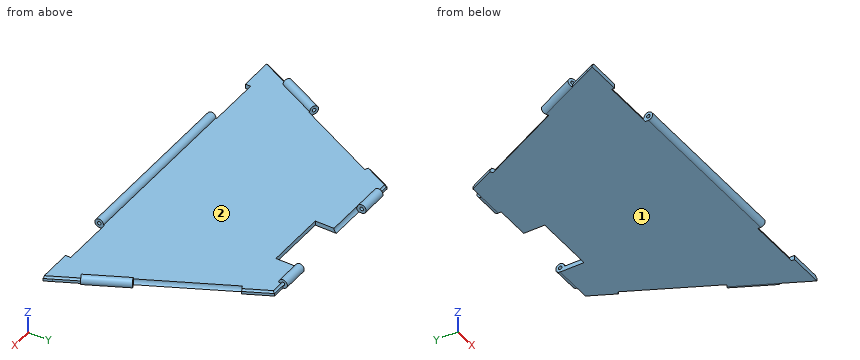
from build123d import *

# Parameters (mm, degrees)
EXTRUDE_1_DEPTH      = 5
SKETCH_9_W           = 30
SKETCH_9_H           = 5
SKETCH_10_R          = 2
CUT_EXTRUDE_3_DEPTH  = 352.212186577
SKETCH_4_W           = 5
SKETCH_4_H           = 50
SKETCH_11_R          = 2
CUT_EXTRUDE_4_DEPTH  = 338.069639722
SKETCH_12_R          = 6
CUT_EXTRUDE_5_DEPTH  = 105
SKETCH_14_R          = 6
CUT_EXTRUDE_6_DEPTH  = 110
SKETCH_3_W           = 200
SKETCH_3_H           = 5
SKETCH_15_R          = 2
CUT_EXTRUDE_7_DEPTH  = 200
SKETCH_16_R          = 6
CUT_EXTRUDE_8_DEPTH  = 60
CUT_EXTRUDE_START    = 60
SKETCH_17_R          = 6
CUT_EXTRUDE_9_DEPTH  = 60
SCALE_1_SCALE        = 0.5
SKETCH_19_W          = 35
SKETCH_19_H          = 12
CUT_EXTRUDE_11_DEPTH = 10


with BuildPart() as part:
    # 草图2 → 凸台-拉伸1 (new body)
    with BuildSketch(Plane(origin=(0, 65.305030884, 0), x_dir=(1, 0, 0), z_dir=(0, 0, 1))):
        Polygon((-200, 0), (-155, 0), (-105, 0), (105, 0), (155, 0), (200, 0), (195.839393539, 8.321212923), (151.118033989, 97.763932023), (100, 200), (50, 200), (-50, 200), (-100, 200), (-151.118033989, 97.763932023), (-195.839393539, 8.321212923), align=None)
    extrude(amount=EXTRUDE_1_DEPTH)

    # 草图9 → 旋转1 (revolve)
    with BuildSketch(Plane(origin=(0, 65.305030884, 5), x_dir=(1, 0, 0), z_dir=(0, 0, 1))):
        with Locations((-70, 197.5)):
            Rectangle(SKETCH_9_W, SKETCH_9_H)
    revolve_1 = revolve(axis=Axis((-85, 265.305030884, 5), (1, 0, 0)))

    # 草图10 → 切除-拉伸3 (cut, symmetric)
    with BuildSketch(Plane(origin=(-85, 65.305030884, 0), x_dir=(0, 0, 1), z_dir=(-1, 0, 0))):
        with Locations(Location((5, 200, 0), (0, 0, 270))):
            Circle(SKETCH_10_R)
    cut_extrude_3 = extrude(amount=CUT_EXTRUDE_3_DEPTH, both=True, mode=Mode.SUBTRACT)

    # 镜向2: 旋转1, 切除-拉伸3 across plane
    add(revolve_1.mirror(Plane(origin=(0, 0, 0), x_dir=(0, 0, 1), z_dir=(1, 0, 0))))
    add(cut_extrude_3.mirror(Plane(origin=(0, 0, 0), x_dir=(0, 0, 1), z_dir=(1, 0, 0))), mode=Mode.SUBTRACT)

    # 草图4 → 旋转2 (revolve)
    with BuildSketch(Plane(origin=(-160, 145.305030884, 0), x_dir=(0, 0, 1), z_dir=(-0.8944271909999162, 0.4472135954999576, 0))):
        with Locations((2.5, -27.639320225)):
            Rectangle(SKETCH_4_W, SKETCH_4_H)
    revolve_2 = revolve(axis=Axis((-161.180339887, 142.944351109, 5), (-0.4472135954999577, -0.894427190999916, 0)))

    # 草图11 → 切除-拉伸4 (cut, symmetric)
    with BuildSketch(Plane(origin=(-23.541019662, 18.222991559, 0), x_dir=(0.8944271909999161, -0.4472135954999577, 0), z_dir=(-0.4472135954999577, -0.8944271909999161, 0))):
        with Locations((-178.8854382, 5)):
            Circle(SKETCH_11_R)
    cut_extrude_4 = extrude(amount=CUT_EXTRUDE_4_DEPTH, both=True, mode=Mode.SUBTRACT)

    # 草图12 → 切除-拉伸5 (cut)
    with BuildSketch(Plane(origin=(-1.180339887, 62.944351109, 0), x_dir=(0.8944271909999161, -0.4472135954999577, 0), z_dir=(0.4472135954999577, 0.8944271909999161, 0))):
        with Locations((-178.8854382, -5)):
            Circle(SKETCH_12_R)
    cut_extrude_5 = extrude(amount=CUT_EXTRUDE_5_DEPTH, mode=Mode.SUBTRACT)

    # 草图14 → 切除-拉伸6 (cut)
    # profile 1 of 2: a face of its own
    with BuildSketch(Plane(origin=(-55, 65.305030884, 0), x_dir=(0, 0, -1), z_dir=(1, 0, 0))):
        with Locations((-5, 200)):
            Circle(SKETCH_14_R)
        with BuildLine():
            Line((-5, 195), (-5, 198))
            ThreePointArc((-5, 198), (-6.414213562, 201.414213562), (-3, 200))
            Line((-3, 200), (0, 200))
            ThreePointArc((0, 200), (-8.535533906, 203.535533906), (-5, 195))
        make_face(mode=Mode.SUBTRACT)
    # profile 2 of 2: a face of its own
    with BuildSketch(Plane(origin=(-55, 65.305030884, 0), x_dir=(0, 0, -1), z_dir=(1, 0, 0))):
        with BuildLine():
            ThreePointArc((0, 200), (-8.535533906, 203.535533906), (-5, 195))
            Line((-5, 195), (-5, 198))
            ThreePointArc((-5, 198), (-6.414213562, 201.414213562), (-3, 200))
            Line((-3, 200), (0, 200))
        make_face()
    extrude(amount=CUT_EXTRUDE_6_DEPTH, mode=Mode.SUBTRACT)

    # 镜向3: 旋转2, 切除-拉伸4, 切除-拉伸5 across plane
    add(revolve_2.mirror(Plane(origin=(0, 0, 0), x_dir=(0, 0, 1), z_dir=(1, 0, 0))))
    add(cut_extrude_4.mirror(Plane(origin=(0, 0, 0), x_dir=(0, 0, 1), z_dir=(1, 0, 0))), mode=Mode.SUBTRACT)
    add(cut_extrude_5.mirror(Plane(origin=(0, 0, 0), x_dir=(0, 0, 1), z_dir=(1, 0, 0))), mode=Mode.SUBTRACT)

    # 草图3 → 旋转3 (revolve)
    with BuildSketch(Plane.XZ.offset(-65.305030884)):
        with Locations((0, 2.5)):
            Rectangle(SKETCH_3_W, SKETCH_3_H)
    revolve(axis=Axis((-100, 65.305030884, 5), (1, 0, 0)))

    # 草图15 → 切除-拉伸7 (cut)
    with BuildSketch(Plane(origin=(100, 65.305030884, 0), x_dir=(0, 0, -1), z_dir=(1, 0, 0))):
        with Locations(Location((-5, 0, 0), (0, 0, 90))):
            Circle(SKETCH_15_R)
    extrude(amount=-CUT_EXTRUDE_7_DEPTH, mode=Mode.SUBTRACT)

    # 草图16 → 切除-拉伸8 (cut)
    with BuildSketch(Plane(origin=(100, 65.305030884, 0), x_dir=(0, 0, -1), z_dir=(1, 0, 0))):
        with Locations((-5, 0)):
            Circle(SKETCH_16_R)
    extrude(amount=CUT_EXTRUDE_8_DEPTH, mode=Mode.SUBTRACT)

    # 草图17 → 切除-拉伸9 (cut)
    with BuildSketch(Plane(origin=(-100, 65.305030884, 0), x_dir=(0, 0, 1), z_dir=(-1, 0, 0)).offset(CUT_EXTRUDE_START)):
        with Locations((5, 0)):
            Circle(SKETCH_17_R)
    extrude(amount=-CUT_EXTRUDE_9_DEPTH, mode=Mode.SUBTRACT)


with BuildPart() as part_1:
    # 缩放比例1: scaled about (0, 0, 0)
    add(part.part.scale(SCALE_1_SCALE))

    # 草图19 → 切除-拉伸11 (cut)
    with BuildSketch(Plane(origin=(0, 0, 0), x_dir=(-1, 0, 0), z_dir=(0, 0, -1))):
        with Locations((-10, 124.994203047)):
            Rectangle(SKETCH_19_W, SKETCH_19_H)
    extrude(amount=-CUT_EXTRUDE_11_DEPTH, mode=Mode.SUBTRACT)


solid = part_1.part
CAD build for the part. Positions are in the model's coordinates, mm. Face numbers are marked on the shaded views. Coordinates: 2 decimals unless noted, no trailing zeros. Loops run counter-clockwise (first coordinate to the right, second up) from the corner with the lowest first, then second, coordinate; pieces in that order, holes last. Notation, with made-up numbers: (31.5, 27.25) -> (47.5, 27.25) arc R22 cw to (47.5, 38.25) -> close; hole circle Ø2 at (87.5, 49). An arc over 180 degrees is marked (long way). One line per item, written item: value.
1. Drill centre lines: line 1 (X direction, y = 69.5, z = 2.85); line 2 (Z direction, x = -18, y = 80.5); line 3 (X direction, y = 63, z = 3.8). Where is each one in solid material? Low to high. Write a range as [from, to].
Answers:
line 1: x = [-84.34, -82.62], [-80.53, -78.81], [78.81, 80.53], [82.62, 84.34]
line 2: z = [0, 2.5]
line 3: x = [-87.21, -82.44], [82.44, 87.21]
2. Slice it at A-A on x = -12. Write the cut outline in (y, z), and give its area (3 significant figures).
Answers:
outline: (32.65, 0) -> (130.99, 0) arc R3 cw to (129.65, 2.5) -> (35.15, 2.5) arc R2.5 ccw (long way) to start; hole circle Ø2 at (32.65, 2.5)
area: 255 mm^2
3. Pull direction X, two halves, no side cores. Call the marked faces 1 and 2: pulls with the +X half, pulls with the -X half, needs draft (parallel to the pull), parting line crosses it, or undercut.
Answers:
face 1: needs draft
face 2: undercut
4. Flat gauge pins, fed straight in: P1, Ø1.2, axis at x = -93.5, z = 1.5, coming from the -Y side; P2, Ø10, axis at x = -68, y = 53.5, coming from the -Z side; P3, Ø1.5, axis at y = 123.5, z = 1.5, coming from the -X side; P4, Ø6, axis at x = 67, y = 44, coming from the +Z side. Where does each tip first touch, or does it go through?
Answers:
P1: stops at y = 32.65
P2: stops at z = 0
P3: stops at x = -54.95
P4: stops at z = 2.5
5. Slice it at C-C on y = 54. Give the number of separate pieces and of enclosed holes in the cut face, and give its area (3 significant figures).
Answers:
separate pieces: 1
enclosed holes: 2
area: 473 mm^2
6. Slice it at B-B on x = 17. Write the cut outline in (y, z).
Answers:
outline: (32.65, 0) -> (118.99, 0) -> (118.99, 2.5) -> (35.15, 2.5) arc R2.5 ccw (long way) to start; hole circle Ø2 at (32.65, 2.5)
